Autodesk Fusion 360 part; units mm, degrees
sketch "Boceto2" plane through (0, 0, 0) normal (0, 1, 0) x (1, 0, 0)
  line L0 (-36.936, 0) -> (-1061.822, 0)
  line L1 (-1061.822, -600) -> (-36.936, -600)
  line L2 (-1008.5735, -150) -> (-650, -150)
  line L3 (-650, -450) -> (-1008.5735, -450)
  arc A0 (-1078.675, -569.2308) -> (-1027.4745, -463.4615) centre (-1500, -300) ccw
  arc A1 (-1027.4745, -136.5385) -> (-1078.675, -30.7692) centre (-1500, -300) ccw
  arc A2 (-650, -450) -> (-500, -300) centre (-650, -300) ccw
  arc A3 (-500, -300) -> (-650, -150) centre (-650, -300) ccw
  circle A4 centre (-410, -300) radius 45
  circle A5 centre (-230, -300) radius 45
  arc A6 (-19.821, -30.3477) -> (-19.821, -569.6523) centre (426.1842, -300) ccw
  arc A7 (-1078.675, -569.2308) -> (-1061.822, -600) centre (-1061.822, -580) ccw
  arc A8 (-36.936, -600) -> (-19.821, -569.6523) centre (-36.936, -580) ccw
  arc A9 (-19.821, -30.3477) -> (-36.936, 0) centre (-36.936, -20) ccw
  arc A10 (-1061.822, 0) -> (-1078.675, -30.7692) centre (-1061.822, -20) ccw
  arc A11 (-1027.4745, -136.5385) -> (-1008.5735, -150) centre (-1008.5735, -130) ccw
  arc A12 (-1008.5735, -450) -> (-1027.4745, -463.4615) centre (-1008.5735, -470) ccw
  point P0 (-1100, 0)
  point P1 (0, -600)
  point P2 (-500, -150)
  point P3 (-500, -450)
  dimension "d1" = 1100
  dimension "d2" = 600
  dimension "d6" = 300
  dimension "d13" = 150
  dimension "d14" = 150
  dimension "d15" = 90
  dimension "d16" = 90
  dimension "d17" = 180
  dimension "d18" = 90
  dimension "d20" = 20
  dimension "d21" = 20
  dimension "d22" = 20
  dimension "d23" = 20
  dimension "d24" = 20
  dimension "d25" = 20
extrude "Extruir1" add sketch "Boceto2" along normal blind 400
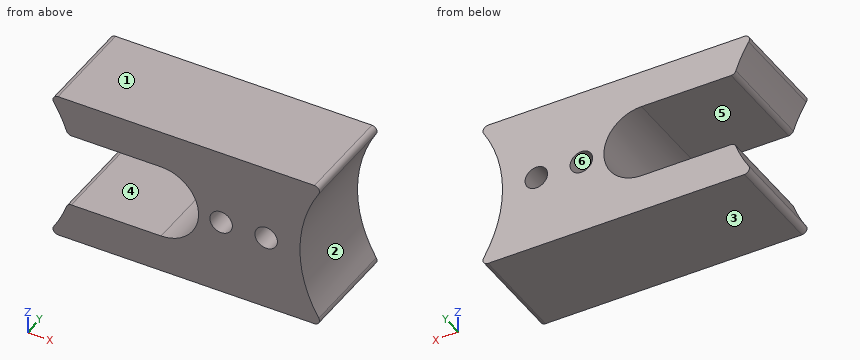
The listing builds one solid part. Answer for the finished solid, in the listing's coordinates (mm). Face numbers are marked on the shaded views. A direction names the side the tool comes from. Give positions to 0.01 mm unless a question says otherwise; leave off trailing zeros. Loops run counter-clockwise (first coordinate to the right, second up) from the corner with the lowest first, then second, coordinate; pieces in that order, holes last. Notation, with made-up numbers: (45.25, 55.5) - (51.25, 55.5) arc R5 ccw to (51.25, 60.5) - close; hole circle Ø8 at (29, -38.75). An arc over 180 degrees is marked (long way). Answer as CSV lines item,"result". Start each with the question number.
Item 1: A cutting plane is placed at C-C on y = 259.5. Determine the outline of the cut face in (x, z) (1 decimal).
Item 2: The mould has two halves that part along Z. Classify the marked faces 1, 2, 3 and 4: +Z half, -Z half, draft (parallel to the pull), parting line (faces both ways), or undercut.
Item 3: A cutting plane is placed at A-A on x = -230. Determine the outline of the cut face in (y, z), then the cut area to 3 significant figures.
Item 4: A cutting plane is placed at B-B on z = 300. Determine the outline of the cut face in (x, y).
Item 5: Each of these flat-tipped pins is pushed along its axis until it touches: pin 1 (8 mm diameter, centred on y = 235.5, z = 318, fed in from +X); pin 2 (3 mm diameter, centred on x = -484, z = 415, fed in from -Y); pin 3 (6 mm diameter, centred on y = 345.5, z = 144.5, fed in from +X). Where does it stop, or does it pass through?
Item 6: A cutting plane is placed at D-D on x = -929.5. Determine the outline of the cut face in (y, z).
Item 7: For the marked faces 5 and 6, determine the directions among +Z, -Z, +X, -X, +Y, -Y from which every point of the face is accessible in a straight line to the end or side of a thin tool.
Item 8: Find the intervals of material crossed by line 1 (X direction, y = 301, z = 300); line 2 (Z direction, x = -993.5, y = 316.5); line 3 (X direction, y = 345, z = 278.5), in increasing order. Write a range as from..to.
Found:
1,outline,"(-1078.7, 30.8) arc R20 ccw to (-1061.8, 0) - (-36.9, 0) arc R20 ccw to (-19.8, 30.3) arc R521.2 cw to (-19.8, 569.7) arc R20 ccw to (-36.9, 600) - (-1061.8, 600) arc R20 ccw to (-1078.7, 569.2) arc R500 cw to (-1027.5, 463.5) arc R20 ccw to (-1008.6, 450) - (-650, 450) arc R150 cw to (-650, 150) - (-1008.6, 150) arc R20 ccw to (-1027.5, 136.5) arc R500 cw to start; hole circle Ø90 at (-410, 300); hole circle Ø90 at (-230, 300)"
2,face 1,"+Z half"
2,face 2,"undercut"
2,face 3,"-Z half"
2,face 4,"undercut"
3,outline,"(0, 0) - (400, 0) - (400, 255) - (0, 255) - close; (0, 345) - (400, 345) - (400, 600) - (0, 600) - close"
3,area,"204,000 mm^2"
4,outline,"(-500, 0) - (-455, 0) - (-455, 400) - (-500, 400) - close; (-365, 0) - (-275, 0) - (-275, 400) - (-365, 400) - close; (-185, 0) - (-95, 0) - (-95, 400) - (-185, 400) - close"
5,pin 1,"stops at x = -94.54"
5,pin 2,"stops at y = 0"
5,pin 3,"stops at x = -70.31"
6,outline,"(0, 0) - (400, 0) - (400, 150) - (0, 150) - close; (0, 450) - (400, 450) - (400, 600) - (0, 600) - close"
7,face 5,"-X, +Y, -Y"
7,face 6,"+Y, -Y"
8,line 1,"x = -500..-455, -365..-275, -185..-95"
8,line 2,"z = 0..150, 450..600"
8,line 3,"x = -501.55..-449.53, -370.47..-269.53, -190.47..-94.56"
